```python
from build123d import *

# Parameters (mm, degrees)
SKETCH1_R           = 2.55
BOSS_EXTRUDE1_DEPTH = 3


with BuildPart() as part:
    # Sketch1 → Boss-Extrude1 (new body)
    with BuildSketch(Plane(origin=(0, 0, 0), x_dir=(1, 0, 0), z_dir=(0, 1, 0))):
        with BuildLine():
            Line((-55, 27.5), (-55, -27.5))
            ThreePointArc((-55, -27.5), (-65, -37.5), (-55, -47.5))
            Line((-55, -47.5), (-55, -98.5))
            Line((-55, -98.5), (55, -98.5))
            Line((55, -98.5), (55, -47.5))
            ThreePointArc((55, -47.5), (65, -37.5), (55, -27.5))
            Line((55, -27.5), (55, 27.5))
            ThreePointArc((55, 27.5), (65, 37.5), (55, 47.5))
            Line((55, 47.5), (55, 98.5))
            Line((55, 98.5), (-55, 98.5))
            Line((-55, 98.5), (-55, 47.5))
            ThreePointArc((-55, 47.5), (-65, 37.5), (-55, 27.5))
        make_face()
        with Locations(Location((-55, 37.5, 0), (0, 0, 270))):
            Circle(SKETCH1_R, mode=Mode.SUBTRACT)
        with Locations(Location((55, 37.5, 0), (0, 0, 270))):
            Circle(SKETCH1_R, mode=Mode.SUBTRACT)
        with Locations(Location((-55, -37.5, 0), (0, 0, 270))):
            Circle(SKETCH1_R, mode=Mode.SUBTRACT)
        with Locations(Location((55, -37.5, 0), (0, 0, 270))):
            Circle(SKETCH1_R, mode=Mode.SUBTRACT)
    extrude(amount=BOSS_EXTRUDE1_DEPTH)


solid = part.part
```
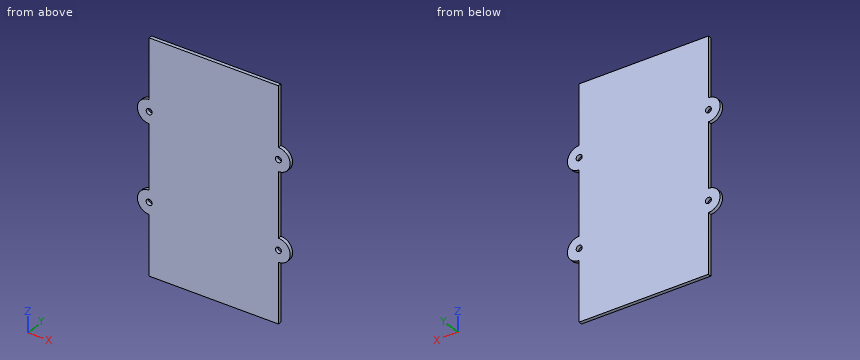
Here's how the part is built. I have some questions about the finished solid (model axes, mm). Round coordinates to 2 decimals unless told otherwise and drop trailing zeros. Order: outer loops, then holes, each group sorted by start corner. A loop starts at its lowest first (then second) coordinate and runs counter-clockwise, first axis right, second up. Notation, with made-up numbers: (0.25, 12.5) -> (4.25, 12.5) arc R8 ccw to (4.25, 22.5) -> close; hole circle Ø7 at (15.25, 11.25). An arc over 180 degrees is marked (long way). Use a Markdown table: item, result. Add a question column.
(1) I need wall thicknesses on line 1 along X through (y, z) = (0.65, -37.5); line 2 along X through (y, z) = (1.1, 62); line 3 along X through (y, z) = (2.7, 30). Which ranges of each line are inside material? Lowest first, please.
(2) Suppose I cut it at D-D, the plane z = -1.5. Please give me the cut outline in (x, y).
(3) Suppose I cut it at A-A, the plane z = -37.5. Please give me the cut outline in (x, y), and give its area (3 significant figures).
(4) Suppose I cut it at C-C, the plane z = 38. Please give me the cut outline in (x, y).
(5) Suppose I cut it at B-B, the plane y = 2.5. Please give me the cut outline in (x, z), and give its area (3 significant figures).
(6) For pin 1 Ø0.9 at (y, z) = (1, 71) entering from -X; pin 2 Ø1.5 at (y, z) = (2, 63.5) entering from +X, each with a flat end and sliding along its axis, tell me the tip position at first contact or that it passes through.
Verdict:
| question | item | result |
|---|---|---|
| 1 | line 1 | -65 to -57.55, -52.45 to 52.45, 57.55 to 65 |
| 1 | line 2 | -55 to 55 |
| 1 | line 3 | -61.61 to 61.61 |
| 2 | outline | (-55, 0) -> (55, 0) -> (55, 3) -> (-55, 3) -> close |
| 3 | outline | (-65, 0) -> (-57.55, 0) -> (-57.55, 3) -> (-65, 3) -> close; (-52.45, 0) -> (52.45, 0) -> (52.45, 3) -> (-52.45, 3) -> close; (57.55, 0) -> (65, 0) -> (65, 3) -> (57.55, 3) -> close |
| 3 | area | 359 mm2 |
| 4 | outline | (-64.99, 0) -> (-57.5, 0) -> (-57.5, 3) -> (-64.99, 3) -> close; (-52.5, 0) -> (52.5, 0) -> (52.5, 3) -> (-52.5, 3) -> close; (57.5, 0) -> (64.99, 0) -> (64.99, 3) -> (57.5, 3) -> close |
| 5 | outline | (-55, -98.5) -> (55, -98.5) -> (55, -47.5) arc R10 ccw to (55, -27.5) -> (55, 27.5) arc R10 ccw to (55, 47.5) -> (55, 98.5) -> (-55, 98.5) -> (-55, 47.5) arc R10 ccw to (-55, 27.5) -> (-55, -27.5) arc R10 ccw to (-55, -47.5) -> close; hole circle Ø5.1 at (-55, -37.5); hole circle Ø5.1 at (-55, 37.5); hole circle Ø5.1 at (55, -37.5); hole circle Ø5.1 at (55, 37.5) |
| 5 | area | 22,200 mm2 |
| 6 | pin 1 | x = -55 |
| 6 | pin 2 | x = 55 |
